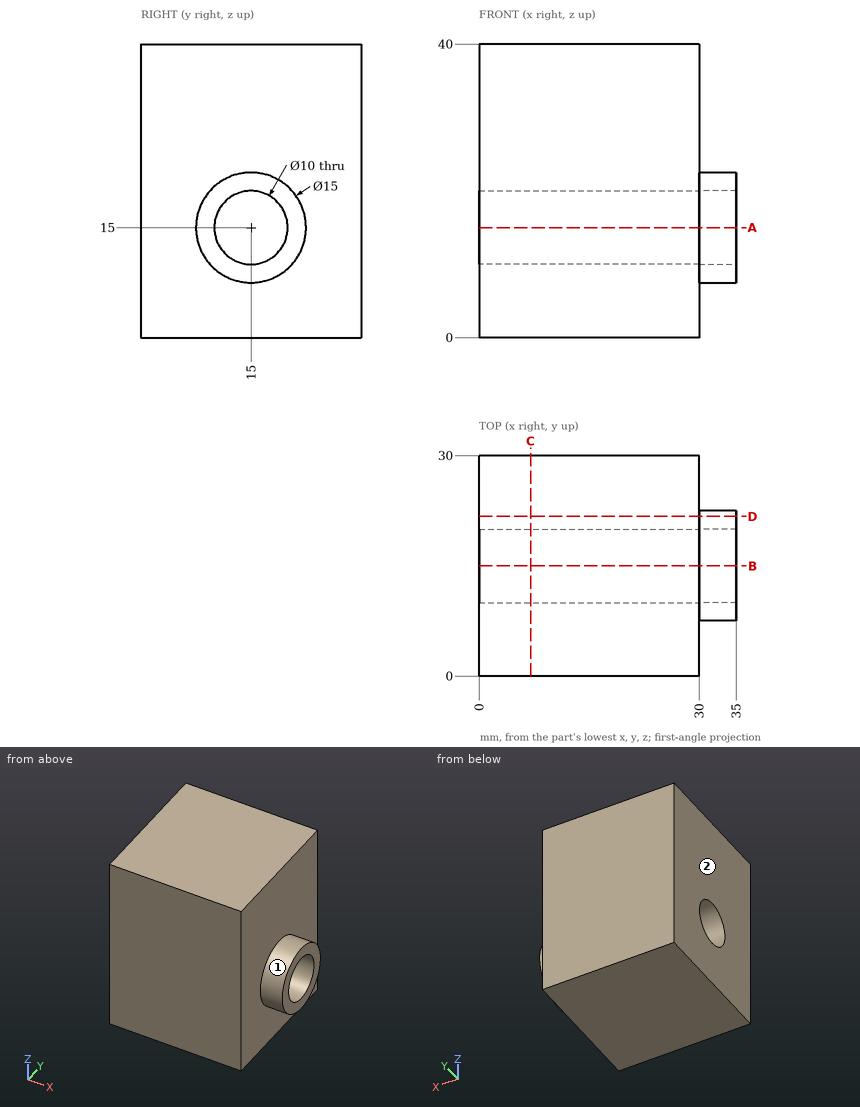
The drawing under review shows one solid part. Ordinate dimensions are in mm from its lowest x, y, z. A direction names the side the tool comes from. Coordinates: 2 decimals unless noted, no trailing zeros. Order: outer loops, then holes, each group sorted by start corner. A loop starts at its lowest first (then second) coordinate and runs counter-clockwise, first axis right, second up. Notation, with made-up numbers: (-1, 4.25) -> (46, 4.25) arc R17 ccw to (46, 15.25) -> close; hole circle Ø11 at (13.25, 1.25). An arc over 180 degrees is marked (long way). Answer in a Markdown table with one row per item.
(1) Consider section A-A (z = 15). Write out the cut boundary in (x, y), plus the area to 3 significant figures.
Answers:
| item | result |
|---|---|
| outline | (0, 0) -> (30, 0) -> (30, 7.5) -> (35, 7.5) -> (35, 10) -> (0, 10) -> close; (0, 20) -> (35, 20) -> (35, 22.5) -> (30, 22.5) -> (30, 30) -> (0, 30) -> close |
| area | 625 mm² |
(2) Machinability: for the marked faces 1 and 2, which of the approach directions +Z, -Z, +X, -X, +Y, -Y give a long, thin tool a straight path to every point of the face, cutting with its end or side? Answer none if there is none.
Answers:
| item | result |
|---|---|
| face 1 | +X |
| face 2 | +Z, -Z, -X, +Y, -Y |
(3) Insertion check: pin 1 (10 mm diameter, centred on x = 22, z = 29, fed in from -Y); pin 2 (4 mm diameter, centred on y = 27, z = 10.5, fed in from +X). Each pin has a flat end and moves straight along its axis. Give the tip position at first contact, or say it passes through.
Answers:
| item | result |
|---|---|
| pin 1 | y = 0 |
| pin 2 | x = 30 |
(4) Consider section B-B (y = 15). Write out the cut boundary in (x, z).
Answers:
| item | result |
|---|---|
| outline | (0, 0) -> (30, 0) -> (30, 7.5) -> (35, 7.5) -> (35, 10) -> (0, 10) -> close; (0, 20) -> (35, 20) -> (35, 22.5) -> (30, 22.5) -> (30, 40) -> (0, 40) -> close |
(5) Consider section C-C (x = 7). Write out the cut boundary in (y, z).
Answers:
| item | result |
|---|---|
| outline | (0, 0) -> (30, 0) -> (30, 40) -> (0, 40) -> close; hole circle Ø10 at (15, 15) |
(6) Consider section D-D (y = 21.75). Write out the cut boundary in (x, z).
Answers:
| item | result |
|---|---|
| outline | (0, 0) -> (30, 0) -> (30, 11.73) -> (35, 11.73) -> (35, 18.27) -> (30, 18.27) -> (30, 40) -> (0, 40) -> close |
(7) Wall thickness on line 1 along Y through (x, z) = (13.75, 15); line 2 along X through (y, z) = (21.5, 9.5); line 3 along Y through (x, z) = (32.7, 15): over which ranges is each line inside the solid? List them lowest first.
Answers:
| item | result |
|---|---|
| line 1 | 0 to 10, 20 to 30 |
| line 2 | 0 to 30 |
| line 3 | 7.5 to 10, 20 to 22.5 |
